from build123d import *

# Parameters (mm, degrees)
F0_W       = 86.36
F0_H       = 6.35
F1_DEPTH   = 19.05
F2_W       = 86.36
F2_H       = 19.05
F2_H_2     = 6.35
F3_DEPTH   = 6.35
F1_FACE1_W = 86.36
F1_FACE1_H = 19.05
F3_FACE_W  = 86.36
F3_FACE_H  = 6.35
F5_R       = 15.24
F6_T       = -2.54
F7_W       = 81.28
F7_H       = 3.81
F8_DEPTH   = 25.4010001


with BuildPart() as f1:
    # F0 (on Front) → F1 (new body)
    with BuildSketch(Plane.XZ):
        Rectangle(F0_W, F0_H)
    extrude(amount=F1_DEPTH)

    # F2 (on face) → F3 (join)
    with BuildSketch(Plane.XZ.offset(19.05)):
        with Locations((0, 12.7)):
            Rectangle(F2_W, F2_H)
        Rectangle(F2_W, F2_H_2)
    extrude(amount=F3_DEPTH)

    # F1_face1 (on face) → F4 section 0
    with BuildSketch(Plane(origin=(0, -9.525, 3.175), x_dir=(1, 0, 0), z_dir=(0, 0, 1))):
        Rectangle(F1_FACE1_W, F1_FACE1_H)
    # F3_face (on face) → F4 section 1
    with BuildSketch(Plane(origin=(0, -22.225, 22.225), x_dir=(1, 0, 0), z_dir=(0, 0, 1))):
        Rectangle(F3_FACE_W, F3_FACE_H)
    loft()

    # F5
    f5_edges = [f1.edges().sort_by_distance(p)[0] for p in [
        (0, -19.05, 22.225),
    ]]
    fillet(f5_edges, radius=F5_R)

    # F6
    f6_openings = [f1.faces().sort_by_distance(p)[0] for p in [
        (0, -25.4, 9.525),
    ]]
    offset(amount=F6_T, openings=f6_openings)

    # F7 (on face) → F8 (cut, through all)
    with BuildSketch(Plane(origin=(0, 0, 0), x_dir=(-1, 0, 0), z_dir=(0, 1, 0))):
        Rectangle(F7_W, F7_H)
    extrude(amount=-F8_DEPTH, mode=Mode.SUBTRACT)


solid = f1.part
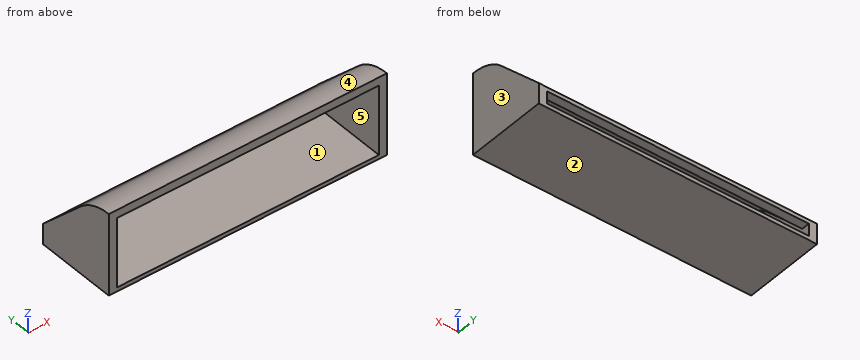
Geometry check sheet. Reference: the model listing, model coordinates, mm. Face numbers are marked on the shaded views. A direction names the side the tool comes from. Coordinates: 2 decimals unless noted, no trailing zeros. Loops run counter-clockwise (first coordinate to the right, second up) from the corner with the lowest first, then second, coordinate; pieces in that order, holes last. Notation, with made-up numbers: (-37.75, 5) - (-27.75, 5) arc R31 cw to (-27.75, 38) - close; hole circle Ø11 at (16, -27.5). An arc over 180 degrees is marked (long way). Use one line per item in the form item = value. Start each with the question number.
Item 1: Gauge pin test, flat end, axial feed: pin 1 (6 mm diameter, centred on x = 0.5, y = -18.5, fed in from +Z). Record the tip position at first contact, or that the pin passes through.
Item 2: Mould release check, pull along Z, two halves, no side actions. Record for the marked faces 3, 4 and 5: +Z half, -Z half, draft (parallel to the pull), parting line (faces both ways), or undercut.
Item 3: Section check B-B, the plane x = -27. Enter the section's corners in (y, z) (3 decimals), and give its area (3 significant figures).
Item 4: Section check A-A, the plane z = 0.75. Enter the section's corners in (x, y), and give its area (3 significant figures).
Item 5: Section check C-C, the plane y = -8. Enter the section's corners in (x, z) (3 decimals).
Item 6: Tool access check on the marked faces 1 and 2. Record the directions out of +Z, -Z, +X, -X, +Y, -Y that give a thin tool (end or side, any length) a straight path to the whole face; none if there is none.
Item 7: Section check D-D, the plane z = 10.5. Enter the section's corners in (x, y) (3 decimals).
Item 8: Thickness scan on probe 1 along X at (y, z) = (-21, 12.25); probe 2 along Z at (x, y) = (13.5, -6) (3 decimals); probe 3 along Z at (x, y) = (-16.5, -11) (3 decimals). Record the ranges inside material, lowest first.
Computed:
q1.pin_1 = 21.73
q2.face_3 = draft
q2.face_4 = +Z half
q2.face_5 = undercut
q3.outline = (-25.4, -3.175) - (0, -3.175) - (0, -1.905) - (-25.4, -1.905) - close; (-25.4, 19.685) - (-25.363, 19.685) arc R12.7 cw to (-16.382, 15.965) - (-2.54, 2.123) - (-2.54, 1.905) - (0, 1.905) - (0, 3.175) - (-14.586, 17.761) arc R15.24 ccw to (-25.363, 22.225) - (-25.4, 22.225) - close
q3.area = 113 mm2
q4.outline = (-43.18, -25.4) - (-40.64, -25.4) - (-40.64, 0) - (-43.18, 0) - close; (40.64, -25.4) - (43.18, -25.4) - (43.18, 0) - (40.64, 0) - close
q4.area = 129 mm2
q5.outline = (-43.18, -3.175) - (43.18, -3.175) - (43.18, 11.175) - (-43.18, 11.175) - close; hole (-40.64, -1.905) - (40.64, -1.905) - (40.64, 7.583) - (-40.64, 7.583) - close
q6.face_1 = +Y, -Y
q6.face_2 = -Z, +X, -X, +Y, -Y
q7.outline = (-43.18, -25.4) - (-40.64, -25.4) - (-40.64, -10.917) - (40.64, -10.917) - (40.64, -25.4) - (43.18, -25.4) - (43.18, -7.325) - (-43.18, -7.325) - close
q8.probe_1 = -43.18 to -40.64, 40.64 to 43.18
q8.probe_2 = -3.175 to -1.905, 5.583 to 9.175
q8.probe_3 = -3.175 to -1.905, 10.583 to 14.175
